The listing builds one solid part. Answer for the finished solid, in the listing's coordinates (mm). A direction names the side the tool comes from. Round coordinates to 2 decimals unless told otherwise and drop trailing zeros. Order: outer loops, then holes, each group sorted by start corner. A loop starts at its lowest first (then second) coordinate and runs counter-clockwise, first axis right, second up. Notation, with made-up numbers: (-2, 43.5) -> (48, 43.5) arc R29 ccw to (48, 74.5) -> close; hole circle Ø6 at (-39, 43.25). An arc over 180 degrees is marked (long way). Answer in a Markdown table with one row per item. Add a question column.
```python
from build123d import *

# Parameters (mm, degrees)
F2_ANGLE = 180
F3_ANGLE = 180
F1_W     = 1.8325150013
F1_H     = 5.3774006665
F1_W_2   = 1.83251407
F1_H_2   = 5.3300224245
F4_DEPTH = 0.25


# Not quite as in the source:
# - ends of sketch curves that miss each other by under 0.0002 mm in the source are joined
# - a feature names something its author has since deleted; it is built from what else it names


with BuildPart() as f2:
    # F0 (on Top) → F2 (revolve)
    with BuildSketch(Plane.XY):
        with BuildLine():
            Line((34.5, 8.2), (34.5, 9.6))
            ThreePointArc((34.5, 9.6), (34.0606601718, 10.6606601718), (33, 11.1))
            Line((33, 11.1), (27.8003929108, 11.1000006409))
            Line((27.8003929108, 11.1000006409), (27.8003929108, 9.600000456))
            Line((27.8003929108, 9.600000456), (23.8003929108, 9.600000456))
            Line((23.8003929108, 9.600000456), (23.8003929108, 11.100000456))
            Line((23.8003929108, 11.100000456), (5.8400444046, 11.0999997705))
            Line((5.8400444046, 11.0999997705), (5.8400444046, 9.6))
            Line((5.8400444046, 9.6), (1.8400444046, 9.6))
            Line((1.8400444046, 9.6), (1.8400444046, 11.1))
            Line((1.8400444046, 11.1), (0, 11.1))
            ThreePointArc((0, 11.1), (-1.0606601718, 10.6606601718), (-1.5, 9.6))
            Line((-1.5, 9.6), (-1.5, 6.9))
            Line((-1.5, 6.9), (0, 6.9))
            Line((0, 6.9), (0, 8.8))
            Line((0, 8.8), (12.2141037136, 8.2))
            Line((12.2141037136, 8.2), (33, 8.2))
            Line((33, 8.2), (33, 6.9))
            Line((33, 6.9), (34.5, 6.9))
            Line((34.5, 6.9), (34.5, 8.2))
        make_face()
    revolve(axis=Axis((17.25, 0, 0), (1, 0, 0)), revolution_arc=F2_ANGLE)



with BuildPart() as f3:
    # F0 (on Top) → F3 (revolve)
    with BuildSketch(Plane.XY):
        with BuildLine():
            Line((34.5, 17.1004687339), (34.5, 18.5004687339))
            Line((34.5, 18.5004687339), (34.5, 19.8004687339))
            Line((34.5, 19.8004687339), (33, 19.8004687339))
            Line((33, 19.8004687339), (33, 18.5004687339))
            Line((33, 18.5004687339), (12.2141037136, 18.5004687339))
            Line((12.2141037136, 18.5004687339), (0, 17.9004687339))
            Line((0, 17.9004687339), (0, 19.8004687339))
            Line((0, 19.8004687339), (-1.5, 19.8004687339))
            Line((-1.5, 19.8004687339), (-1.5, 17.1004687339))
            ThreePointArc((-1.5, 17.1004687339), (-1.0606601718, 16.0398085621), (0, 15.6004687339))
            Line((0, 15.6004687339), (1.8400444046, 15.6004687339))
            Line((1.8400444046, 15.6004687339), (1.8400444046, 17.1004687339))
            Line((1.8400444046, 17.1004687339), (5.8400444046, 17.1004687339))
            Line((5.8400444046, 17.1004687339), (5.8400444046, 15.6004687339))
            Line((5.8400444046, 15.6004687339), (23.8003929108, 15.6004682779))
            Line((23.8003929108, 15.6004682779), (23.8003929108, 17.1004682779))
            Line((23.8003929108, 17.1004682779), (27.8003929108, 17.1004682779))
            Line((27.8003929108, 17.1004682779), (27.8003929108, 15.6004680931))
            Line((27.8003929108, 15.6004680931), (33, 15.6004687339))
            ThreePointArc((33, 15.6004687339), (34.0606601718, 16.0398085621), (34.5, 17.1004687339))
        make_face()
    revolve(axis=Axis((17.25, 26.7004687339, 0), (-1, 0, 0)), revolution_arc=F3_ANGLE)


with BuildPart() as f2_1:
    add(f2.part)

    add(f3.part)  # F4 merges F3
    # F1 (on Top) → F4 (join)
    with BuildSketch(Plane.XY):
        with Locations((30.2449278533, 13.3801726624)):
            Rectangle(F1_W, F1_H)
        with Locations((8.218171075, 13.3564835414)):
            Rectangle(F1_W_2, F1_H_2)
    extrude(amount=F4_DEPTH)


solid = f2_1.part
```
Item 1: The part is cut by section C-C, the plane z = 1.25. State how many separate pieces and enclosed holes the cut face has, and give its area (3 significant figures).
Item 2: Find the intervals of material crossed by probe 1 along Y at (x, z) = (15, 5.25); probe 2 along Y at (x, z) = (7, 7) (3 decimals); probe 3 along X at (y, z) = (-7, 8.5), in increasing order. Write a range as [from, to].
Item 3: For a pull along Y with two mould halves and no side action, classify faces 4 (the face through (30, 13, 0.25)), 5 (the face through (34.5, 29, 7)) as released by +Y, released by -Y, zero draft, split by the parting line, or undercut.
Item 4: The part is cut by section A-A, the plane x = 17. Give the vertices of the cut face in (y, z).
Item 5: Flat-ended cylindrical pins translate along their axes: P1, Ø0.9, axis at x = 30, y = 12.5, coming from the +Z side; P2, Ø5, axis at x = 20.5, y = 22.5, coming from the -Z side. Find the tip coordinate at first contact, or state that the pin passes through.
Item 6: The part is cut by section B-B, the plane y = 0. Give the vertices of the cut face in (x, z), and give its area (3 significant figures).
Item 7: A tool of negligible diameter and unlimited length cuts with its end or side. For faces 1 (the face through (-0.76, 26.55, 6.9)), 2 (the face through (22.46, 26.52, 8.2)), 3 (the face through (5.84, 1, 10)), from which of +Z, -Z, +X, -X, +Y, -Y can it reach the whole face along a straight path? Write none if from no direction.
Resolved:
| question | item | result |
|---|---|---|
| 1 | separate pieces | 4 |
| 1 | enclosed holes | 0 |
| 1 | area | 370 mm2 |
| 2 | probe 1 | [-9.78, -6.3], [6.3, 9.78], [16.92, 20.4], [33, 36.48] |
| 2 | probe 2 | [-8.615, -4.744], [4.744, 8.615], [18.086, 21.956], [31.445, 35.315] |
| 2 | probe 3 | [-0.51, 1.84], [5.84, 23.8], [27.8, 33.51] |
| 3 | face 4 | undercut |
| 3 | face 5 | zero draft |
| 4 | outline | (-11.1, 0) -> (-8.2, 0) arc R8.2 cw to (8.2, 0) -> (11.1, 0) arc R11.1 ccw to start; (15.6, 0) -> (18.5, 0) arc R8.2 cw to (34.9, 0) -> (37.8, 0) arc R11.1 ccw to start |
| 5 | P1 | z = 0.25 |
| 5 | P2 | z = 4.73 |
| 6 | outline | (-1.5, 6.9) -> (0, 6.9) -> (0, 8.8) -> (12.21, 8.2) -> (33, 8.2) -> (33, 6.9) -> (34.5, 6.9) -> (34.5, 9.6) arc R1.5 ccw to (33, 11.1) -> (27.8, 11.1) -> (27.8, 9.6) -> (23.8, 9.6) -> (23.8, 11.1) -> (5.84, 11.1) -> (5.84, 9.6) -> (1.84, 9.6) -> (1.84, 11.1) -> (0, 11.1) arc R1.5 ccw to (-1.5, 9.6) -> close |
| 6 | area | 91.7 mm2 |
| 7 | face 1 | -Z, +X, -X |
| 7 | face 2 | -Z |
| 7 | face 3 | +Z |
